Check sheet for the modelled part. Datum: model origin and axes. Units: mm. A direction names the side the tool comes from. Give positions to 0.01 mm unless a question says otherwise; leave off trailing zeros. Loops run counter-clockwise (first coordinate to the right, second up) from the corner with the lowest first, then second, coordinate; pieces in that order, holes last. Notation, with made-up numbers: (37.25, 47) -> (82.25, 47) arc R20 cw to (82.25, 75) -> close; hole circle Ø3 at (9.5, -10). An arc over 180 degrees is marked (long way). Write each question's results on one line, items separated by ' | '. Start each with the question number.
1. Gauge pin test, flat ends, axial feed: pin 1 Ø6 at (x, y) = (1, 7) entering from -Z; pin 2 Ø1.5 at (x, y) = (41.5, 2.5) entering from +Z; pin 3 Ø6 at (x, z) = (32, -12.5) entering from +Y; pin 4 Ø2.5 at (x, z) = (-31.18, -20.385) entering from +Y. Record the tip position at first contact, or that the pin passes through.
2. Material ranges on L1, parallel to X at y = 1, z = 23.5; L2, parallel to X at y = 3.5, z = -23; L3, parallel to X at y = 6.75, z = -17.5, recorded low to high. Write a range as from..to.
3. Cross-section at B-B on x = 31.18. Record the boundary of the cut face in (y, z) (3 decimals), and give its area (3 significant figures).
4. Tool access check on faces 1 (the face through (27.63, 2, -21)), 2 (the face through (40.25, 5, -3)), 3 (the face through (37, 4, 3)), 4 (the face through (2, 5, 9.102)), 5 (the face through (2, 10.3, 17)). Record the directions out of +Z, -Z, +X, -X, +Y, -Y that give a thin tool (end or side, any length) a straight path to the whole face; none if there is none.
5. Mould release check, pull along X, two halves, no side actions. Record for faces 6 (the face through (31, 0, -22)), 7 (the face through (17, 2, 28.775)), 8 (the face through (40.398, 7.395, -30.768)): +X half, -X half, draft (parallel to the pull), parting line (faces both ways), or undercut.
6. Cross-section at A-A on z = -14. Record the boundary of the cut face in (x, y).
7. Cross-section at C-C on y = 5.5. Count the separate pieces of the cut face and the enclosed holes in it, and give its area (3 significant figures).
8. Cross-section at D-D on z = 11. Record the boundary of the cut face in (x, y), and give its area (3 significant figures).
from build123d import *

# Parameters (mm, degrees)
SKETCH_2_W          = 70.5
SKETCH_2_H          = 51.55
EXTRUDE_1_DEPTH     = 15
SKETCH_3_W          = 7.62
SKETCH_3_H          = 8.89
SKETCH_3_R          = 1.35
EXTRUDE_2_DEPTH     = 4
SKETCH_4_W          = 47.8178
SKETCH_4_H          = 8
CUT_EXTRUDE_1_DEPTH = 15
SKETCH_5_W          = 5.24256
SKETCH_5_H          = 16.6727
SKETCH_5_W_2        = 6.22916
SKETCH_5_H_2        = 5.01906
EXTRUDE_3_DEPTH     = 10.3
SKETCH_7_W          = 8
SKETCH_7_H          = 12.7
CUT_EXTRUDE_4_DEPTH = 4
CUT_EXTRUDE_5_DEPTH = 2.2
SKETCH_11_W         = 10.60647
SKETCH_11_H         = 8
CUT_EXTRUDE_6_DEPTH = 10
SKETCH_12_W         = 17
SKETCH_12_H         = 3
CUT_EXTRUDE_7_DEPTH = 4


with BuildPart() as part:
    # 草图2 → 凸台-拉伸1 (new body)
    with BuildSketch(Plane(origin=(0, 0, 0), x_dir=(1, 0, 0), z_dir=(0, 1, 0))):
        with BuildLine():
            Line((-33.25, -33.775), (33.25, -33.775))
            ThreePointArc((33.25, -33.775), (40.321067812, -30.846067812), (43.25, -23.775))
            Line((43.25, -23.775), (43.25, 23.775))
            ThreePointArc((43.25, 23.775), (40.321067812, 30.846067812), (33.25, 33.775))
            Line((33.25, 33.775), (-33.25, 33.775))
            ThreePointArc((-33.25, 33.775), (-40.321067812, 30.846067812), (-43.25, 23.775))
            Line((-43.25, 23.775), (-43.25, -23.775))
            ThreePointArc((-43.25, -23.775), (-40.321067812, -30.846067812), (-33.25, -33.775))
        make_face()
        Rectangle(SKETCH_2_W, SKETCH_2_H, mode=Mode.SUBTRACT)
    extrude(amount=EXTRUDE_1_DEPTH)

    # 草图3 → 凸台-拉伸2 (add)
    # profile 1 of 2: a face of its own
    with BuildSketch(Plane(origin=(0, 0, 0), x_dir=(1, 0, 0), z_dir=(0, 1, 0))):
        with Locations((-31.44, 21.33)):
            Rectangle(SKETCH_3_W, SKETCH_3_H)
        with Locations(Location((-31.18, 20.385, 0), (0, 0, 270))):
            Circle(SKETCH_3_R, mode=Mode.SUBTRACT)
    # profile 2 of 2: a face of its own
    with BuildSketch(Plane(origin=(0, 0, 0), x_dir=(1, 0, 0), z_dir=(0, 1, 0))):
        with Locations((31.44, 21.33)):
            Rectangle(SKETCH_3_W, SKETCH_3_H)
        with Locations(Location((31.18, 20.385, 0), (0, 0, 270))):
            Circle(SKETCH_3_R, mode=Mode.SUBTRACT)
    extrude(amount=EXTRUDE_2_DEPTH)

    # 草图4 → 切除-拉伸1 (cut)
    with BuildSketch(Plane(origin=(0, 15, 0), x_dir=(1, 0, 0), z_dir=(0, 1, 0))):
        with Locations((-3.7211, 29.775)):
            Rectangle(SKETCH_4_W, SKETCH_4_H)
    extrude(amount=-CUT_EXTRUDE_1_DEPTH, mode=Mode.SUBTRACT)

    # 草图5 → 凸台-拉伸3 (add)
    with BuildSketch(Plane(origin=(0, 0, 0), x_dir=(1, 0, 0), z_dir=(0, 1, 0))):
        with Locations((2.17558, -17.43865)):
            Rectangle(SKETCH_5_W, SKETCH_5_H)
        with Locations((32.13542, 8.50953)):
            Rectangle(SKETCH_5_W_2, SKETCH_5_H_2)
    extrude(amount=EXTRUDE_3_DEPTH)

    # 草图7 → 切除-拉伸4 (cut)
    with BuildSketch(Plane.XZ):
        with Locations((39.25, 2.91792)):
            Rectangle(SKETCH_7_W, SKETCH_7_H)
    extrude(amount=-CUT_EXTRUDE_4_DEPTH, mode=Mode.SUBTRACT)

    # 草图9 → 切除-拉伸5 (cut)
    with BuildSketch(Plane.ZY.offset(-38.05)):
        Polygon((-23.775, 8), (23.775, 8), (23.775, 0), (-33.775, 0), (-33.775, 4), (-23.775, 4), align=None)
    extrude(amount=-CUT_EXTRUDE_5_DEPTH, mode=Mode.SUBTRACT)

    # 草图11 → 切除-拉伸6 (cut)
    with BuildSketch(Plane(origin=(0, 0, 0), x_dir=(-1, 0, 0), z_dir=(0, -1, 0))):
        with Locations((16.673805, -29.775)):
            Rectangle(SKETCH_11_W, SKETCH_11_H)
    extrude(amount=-CUT_EXTRUDE_6_DEPTH, mode=Mode.SUBTRACT)

    # 草图12 → 切除-拉伸7 (cut)
    with BuildSketch(Plane.XZ):
        with Locations((16.773075079, 27.275)):
            Rectangle(SKETCH_12_W, SKETCH_12_H)
    extrude(amount=-CUT_EXTRUDE_7_DEPTH, mode=Mode.SUBTRACT)


solid = part.part
Geometry says:
1) pin 1: z = 9.1 | pin 2: z = 30.39 | pin 3: y = 10.3 | pin 4: through
2) L1: -43.25..-35.25, -0.45..4.8, 35.25..38.05, 40.25..43.25 | L2: -43.25..-27.63, 27.63..38.05, 40.25..43.25 | L3: -43.25..-35.25, 35.25..38.05, 40.25..43.25
3) outline: (0, -33.775) -> (15, -33.775) -> (15, -25.775) -> (4, -25.775) -> (4, -21.735) -> (0, -21.735) -> close; (0, -19.035) -> (4, -19.035) -> (4, -16.885) -> (0, -16.885) -> close; (0, -11.019) -> (10.3, -11.019) -> (10.3, -6) -> (0, -6) -> close; (0, 25.775) -> (15, 25.775) -> (15, 33.775) -> (0, 33.775) -> close | area: 316 mm^2
4) face 1: +Y, -Y | face 2: -Y | face 3: +X, -Y | face 4: -Z, +Y, -Y | face 5: -Z, +Y
5) face 6: draft | face 7: undercut | face 8: +X half
6) outline: (-43.25, 0) -> (-35.25, 0) -> (-35.25, 15) -> (-43.25, 15) -> close; (35.25, 0) -> (38.05, 0) -> (38.05, 8) -> (40.25, 8) -> (40.25, 0) -> (43.25, 0) -> (43.25, 15) -> (35.25, 15) -> close
7) separate pieces: 2 | enclosed holes: 1 | area: 1,670 mm^2
8) outline: (-43.25, 0) -> (-35.25, 0) -> (-35.25, 15) -> (-43.25, 15) -> close; (-0.45, 0) -> (4.8, 0) -> (4.8, 10.3) -> (-0.45, 10.3) -> close; (35.25, 0) -> (38.05, 0) -> (38.05, 8) -> (40.25, 8) -> (40.25, 0) -> (43.25, 0) -> (43.25, 15) -> (35.25, 15) -> close | area: 276 mm^2
